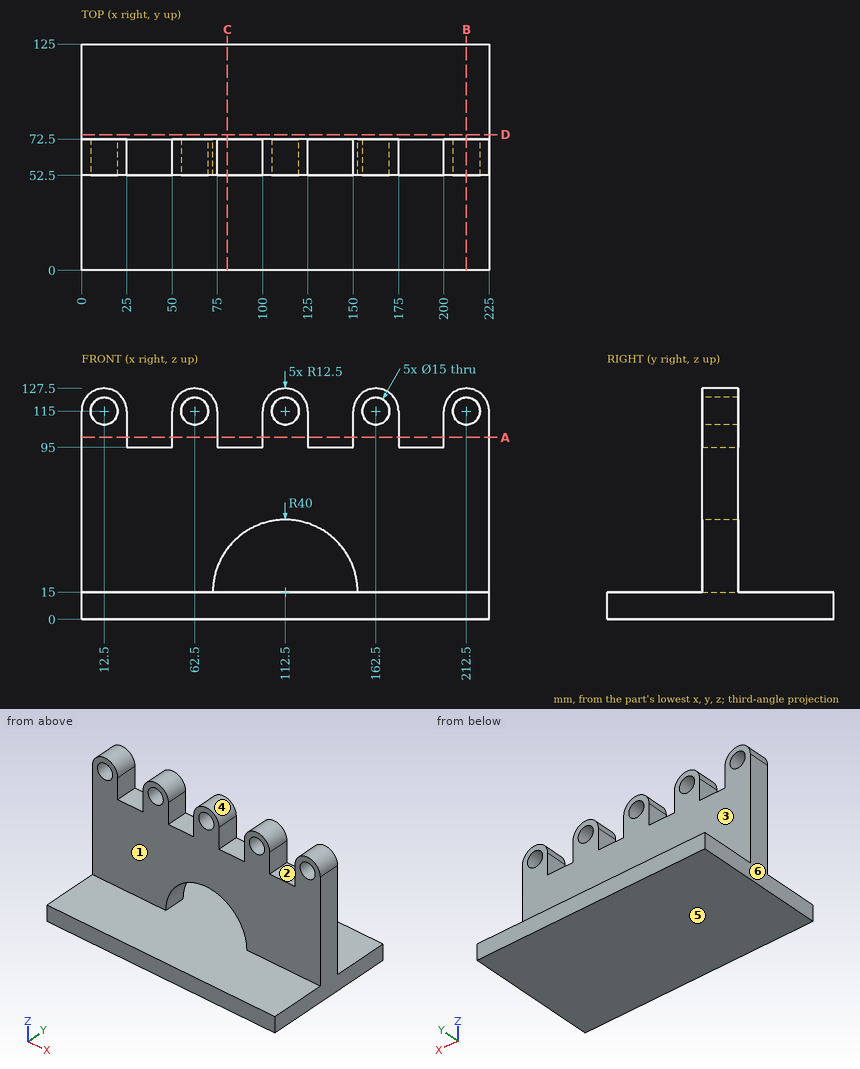
Geometry check sheet. Reference: drawing and pictorial views, mm from the part's lowest x, y, z. A direction names the side the tool comes from. Coordinates: 2 decimals unless noted, no trailing zeros. Order: outer loops, then holes, each group sorted by start corner. A loop starts at its lowest first (then second) coordinate and runs counter-clockwise, first axis right, second up.
1. Sectioned sample at B-B, the plane x = 212.5. Record the cut outline in (y, z).
Results found:
outline: (0, 0) - (125, 0) - (125, 15) - (72.5, 15) - (72.5, 107.5) - (52.5, 107.5) - (52.5, 15) - (0, 15) - close; (52.5, 122.5) - (72.5, 122.5) - (72.5, 127.5) - (52.5, 127.5) - close
2. Sectioned sample at C-C, the plane x = 80.5. Record the cut outline in (y, z).
Results found:
outline: (0, 0) - (125, 0) - (125, 15) - (0, 15) - close; (52.5, 39) - (72.5, 39) - (72.5, 95) - (52.5, 95) - close
3. Set-up check for the marked faces 1, 2 and 3: record each of +Z, -Z, +X, -X, +Y, -Y from which the full face is reachable in a straight line by a thin tool's end or side.
Results found:
face 1: +Z, +X, -X, -Y
face 2: +Z, +Y, -Y
face 3: +Z, +X, -X, +Y
4. Scan lines: line 1 (Z direction, x = 111, y = 10.5); line 2 (Y direction, x = 120.5, z = 107.5); line 3 (Z direction, x = 91, y = 71.5). Record each from-to range of solid material in increasing order.
Results found:
line 1: z = 0 to 15
line 2: y = 52.5 to 72.5
line 3: z = 0 to 15, 48.73 to 95
5. Go/stop test with flat-tipped pins: pin 1 Ø1 at (x, z) = (71, 99.5) entering from -Y; pin 2 Ø22 at (y, z) = (65.5, 105.5) entering from -X; pin 3 Ø1.5 at (x, y) = (68, 41) entering from +Z; pin 4 Ø6 at (x, y) = (40, 58) entering from +Z. Record where each tip stops, or that it passes through.
Results found:
pin 1: stops at y = 52.5
pin 2: stops at x = 0
pin 3: stops at z = 15
pin 4: stops at z = 95
6. Sectioned sample at D-D, the plane y = 75. Record the cut outline in (x, z), and give its area (4 significant figures).
Results found:
outline: (0, 0) - (225, 0) - (225, 15) - (0, 15) - close
area: 3,375 mm2
7. Sectioned sample at A-A, the plane z = 100.5. Record the cut outline in (x, y), and give its area (3 significant figures).
Results found:
outline: (0, 52.5) - (25, 52.5) - (25, 72.5) - (0, 72.5) - close; (50, 52.5) - (75, 52.5) - (75, 72.5) - (50, 72.5) - close; (100, 52.5) - (125, 52.5) - (125, 72.5) - (100, 72.5) - close; (150, 52.5) - (175, 52.5) - (175, 72.5) - (150, 72.5) - close; (200, 52.5) - (225, 52.5) - (225, 72.5) - (200, 72.5) - close
area: 2,500 mm2
8. Release check for a two-part mould opening along X. For the marked faces 4, 5 and 6 record: +X half, -X half, draft (parallel to the pull), parting line (faces both ways), or undercut.
Results found:
face 4: undercut
face 5: draft
face 6: -X half
